Can you work these out from the drawing? Everything is in mm from the part's minimum corner. A direction names the side the tool comes from. Round coordinates to 2 decimals unless told otherwise and drop trailing zeros. Write each loop counter-clockwise with the first axis right and the second up, starting at its lowest first coordinate (ties: lowest second). Pieces come first, ordered by that corner, then holes. Notation, with made-up numbers: M 3,23.5 L 17,23.5 A27 ccw 17,60.5 Z; hole C 76,57.5 d1. An arc over 180 degrees is marked long. Use a Markdown table: item, result. Add a question column.
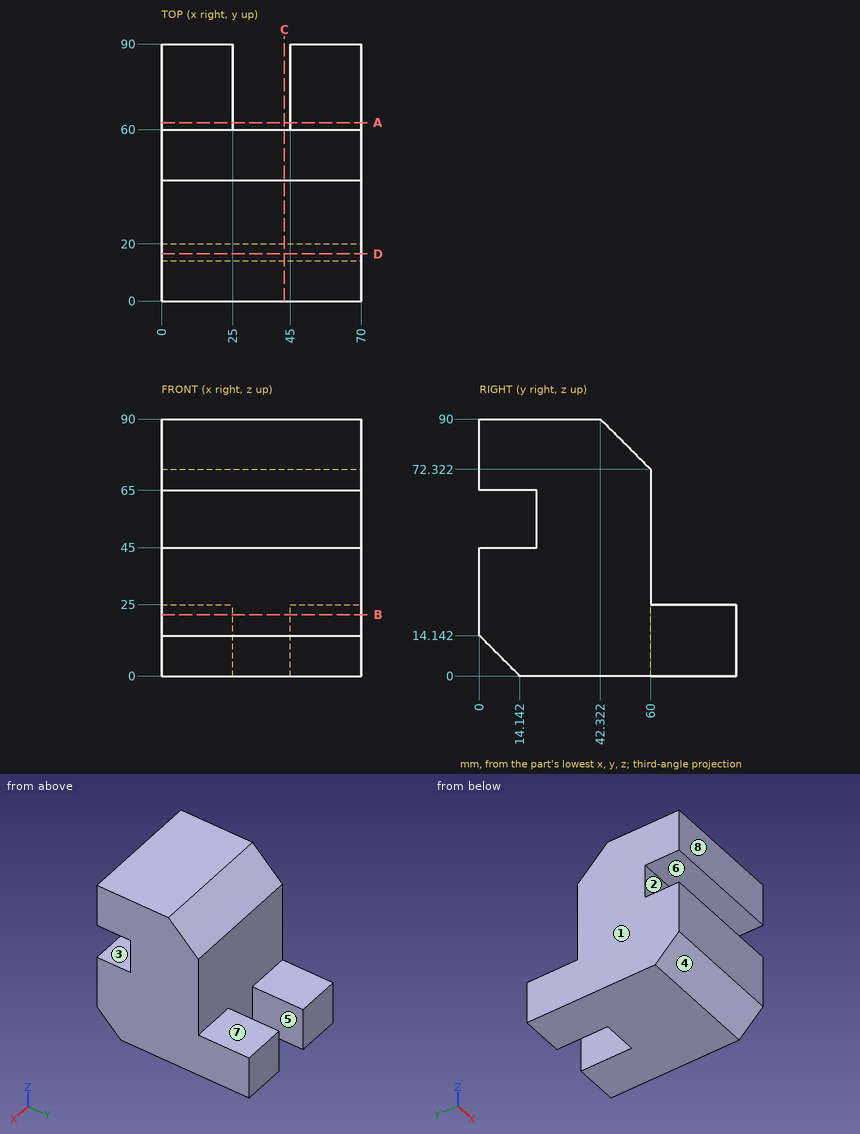
Item 1: Imagine slicing it at A-A on y = 62.5. List the corners of the cut face in (x, z) for me, plus the area to 3 significant figures.
Item 2: If we mould it in two halves opening along Z, with no side actions, what happens to the marked faces 1, 2, 3 and 4? For each: +Z half, -Z half, draft (parallel to the pull), parting line (faces both ways), or undercut.
Item 3: Imagine slicing it at C-C on x = 43. List the corners of the cut face in (y, z) for me, plus the area to 3 significant figures.
Item 4: On a 3-axis mill with a long thin cutter (end or side, diameter ignored), from which of +Z, -Z, +X, -X, +Y, -Y can I reach the whole of each face in a straight line? I mean the marked faces 5, 6, 7 and 8. Say none if no direction works.
Item 5: I need wall thicknesses on probe 1 along X at (y, z) = (84.5, 21); probe 2 along Z at (x, y) = (53, 19.5); probe 3 along Z at (x, y) = (53.5, 62). Which ranges of each line are inside material? Lowest first, please. Write a range as from..to.
Item 6: Imagine slicing it at D-D on y = 16.5. List the corners of the cut face in (x, z) for me.
Item 7: Imagine slicing it at B-B on z = 21.5. List the corners of the cut face in (x, y) for me, plus the area to 3 significant figures.
Item 8: For pin 1 Ø1.5 at (x, y) = (56.5, 75) entering from +Z, with a flat end and sliding along its axis, tell me the tip position at first contact or that it passes through.
The answers:
| question | item | result |
|---|---|---|
| 1 | outline | M 0,0 L 25,0 L 25,25 L 0,25 Z; M 45,0 L 70,0 L 70,25 L 45,25 Z |
| 1 | area | 1,250 mm² |
| 2 | face 1 | draft |
| 2 | face 2 | undercut |
| 2 | face 3 | undercut |
| 2 | face 4 | -Z half |
| 3 | outline | M 0,14.14 L 14.14,0 L 60,0 L 60,72.32 L 42.32,90 L 0,90 L 0,65 L 20,65 L 20,45 L 0,45 Z |
| 3 | area | 4,740 mm² |
| 4 | face 5 | +Z, -Z, +Y |
| 4 | face 6 | +X, -X, -Y |
| 4 | face 7 | +Z, +X, -X, +Y |
| 4 | face 8 | +Z, -Z, +X, -X, -Y |
| 5 | probe 1 | 0..25, 45..70 |
| 5 | probe 2 | 0..45, 65..90 |
| 5 | probe 3 | 0..25 |
| 6 | outline | M 0,0 L 70,0 L 70,45 L 0,45 Z; M 0,65 L 70,65 L 70,90 L 0,90 Z |
| 7 | outline | M 0,0 L 70,0 L 70,90 L 45,90 L 45,60 L 25,60 L 25,90 L 0,90 Z |
| 7 | area | 5,700 mm² |
| 8 | pin 1 | z = 25 |
